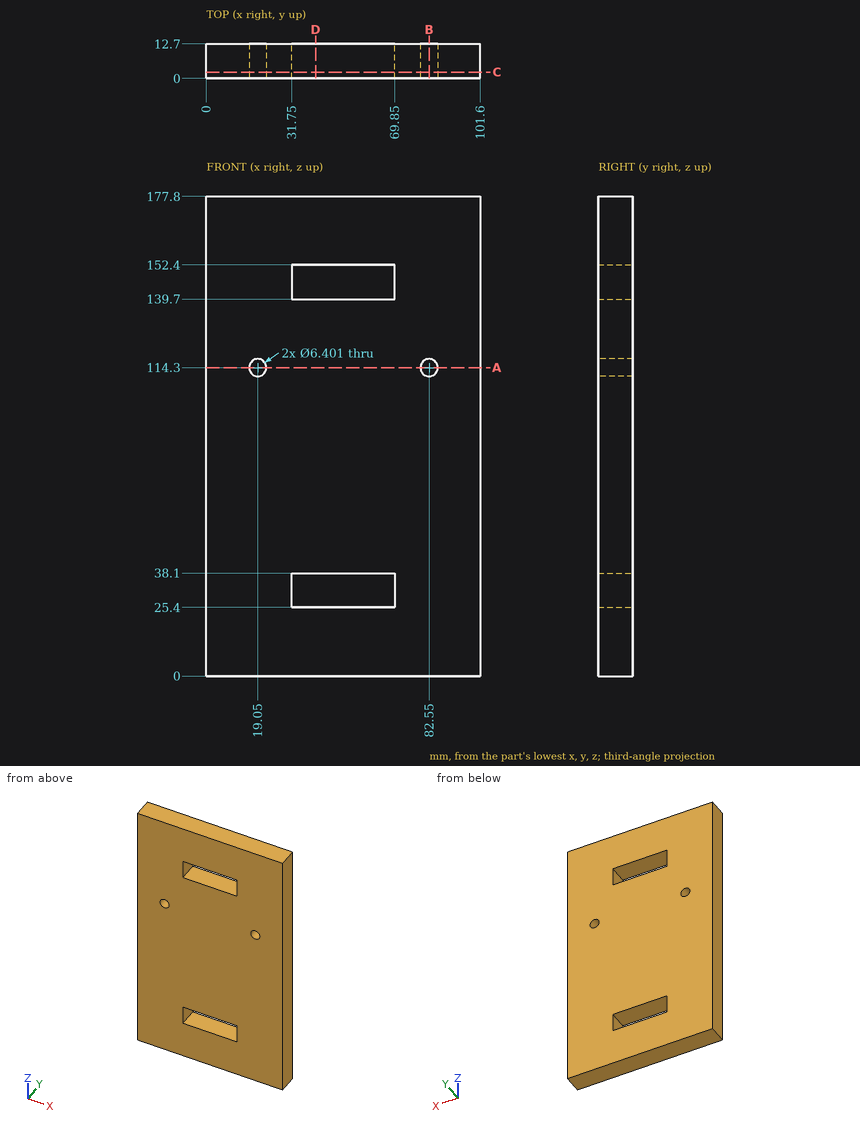
Can you work these out from the drawing? Everything is in mm from the part's minimum corner. Give positions to 0.01 mm unless a question says otherwise; leave off trailing zeros. Write each loop counter-clockwise with the first axis right and the second up, starting at its lowest first coordinate (ties: lowest second). Pieces come first, ordered by that corner, then holes. Notation, with made-up numbers: (-7, -13) -> (48, -13) arc R27 ccw to (48, 19) -> close; hole circle Ø8 at (89, -19). An arc over 180 degrees is marked (long way). Write each question's results on one line, items separated by ' | '. Start each with the question number.
Q1. I need wall thicknesses on probe 1 along Z at (x, y) = (35.5, 3.25); probe 2 along X at (y, z) = (8.75, 114.3); probe 3 along Z at (x, y) = (82.55, 7.75). Which ranges of each line are inside material? Lowest first, please.
Q2. Suppose I cut it at B-B, the plane x = 82.55. List the corners of the cut face in (y, z) for me, and give its area (3 significant figures).
Q3. Suppose I cut it at A-A, the plane z = 114.3. List the corners of the cut face in (x, y) for me.
Q4. Suppose I cut it at C-C, the plane y = 2.25. List the corners of the cut face in (x, z) for me.
Q5. Suppose I cut it at D-D, the plane x = 40.5. List the corners of the cut face in (y, z) for me, and give its area (3 significant figures).
Outcome:
1) probe 1: 0 to 25.4, 38.1 to 139.7, 152.4 to 177.8 | probe 2: 0 to 15.85, 22.25 to 79.35, 85.75 to 101.6 | probe 3: 0 to 111.1, 117.5 to 177.8
2) outline: (0, 0) -> (12.7, 0) -> (12.7, 111.1) -> (0, 111.1) -> close; (0, 117.5) -> (12.7, 117.5) -> (12.7, 177.8) -> (0, 177.8) -> close | area: 2,180 mm2
3) outline: (0, 0) -> (15.85, 0) -> (15.85, 12.7) -> (0, 12.7) -> close; (22.25, 0) -> (79.35, 0) -> (79.35, 12.7) -> (22.25, 12.7) -> close; (85.75, 0) -> (101.6, 0) -> (101.6, 12.7) -> (85.75, 12.7) -> close
4) outline: (0, 0) -> (101.6, 0) -> (101.6, 177.8) -> (0, 177.8) -> close; hole circle Ø6.4 at (19.05, 114.3); hole (31.75, 25.4) -> (69.85, 25.4) -> (69.85, 38.1) -> (31.75, 38.1) -> close; hole (31.75, 139.7) -> (69.85, 139.7) -> (69.85, 152.4) -> (31.75, 152.4) -> close; hole circle Ø6.4 at (82.55, 114.3)
5) outline: (0, 0) -> (12.7, 0) -> (12.7, 25.4) -> (0, 25.4) -> close; (0, 38.1) -> (12.7, 38.1) -> (12.7, 139.7) -> (0, 139.7) -> close; (0, 152.4) -> (12.7, 152.4) -> (12.7, 177.8) -> (0, 177.8) -> close | area: 1,940 mm2
